For this review, take the finished solid that the model builds, in its own axes (mm). Coordinates: 2 decimals unless noted, no trailing zeros. Loops run counter-clockwise (first coordinate to the right, second up) from the corner with the lowest first, then second, coordinate; pieces in that order, holes last.
1. Take a section at B-B, the plane x = -0.2. Count the separate pieces of the cut face and the enclosed holes in it, then the cut area to 3 significant figures.
2. To check wall thickness, follow probe 1 along Z at (x, y) = (0.4, 15); probe 2 along Y at (x, z) = (-0.75, -85); probe 3 along Y at (x, z) = (0.65, -32.5). State the ranges of each line that lie inside material, in increasing order.
3. Take a section at D-D, the plane z = -68. State the section outline as (x, y) points.
4. Take a section at A-A, the plane z = -22. State the section outline as (x, y) points.
5. Take a section at C-C, the plane y = 57.5. State the section outline as (x, z) points.
6. Clearance check with flat-ended pins moving along their axes: P1, Ø2, axis at x = 0, z = -27, coming from the +Y side; P2, Ø1, axis at x = -1.5, y = 49, coming from the +Z side; P3, Ø2.5, axis at y = 15, z = -85, coming from the -X side; P4, Ø2, axis at x = 1, y = 6.5, coming from the +Z side. State where each tip first meets the part, or that it passes through.
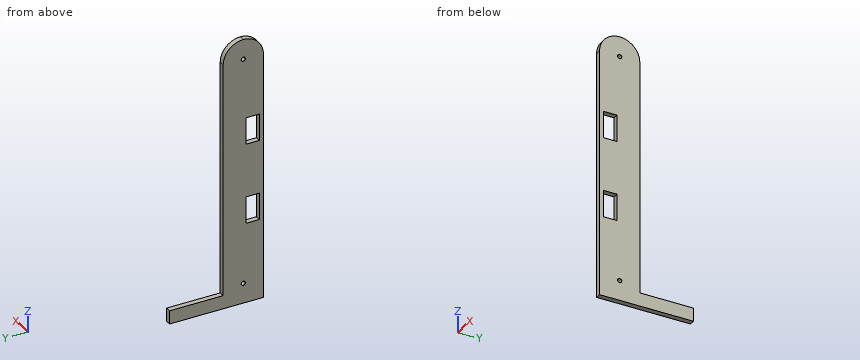
Autodesk Inventor part; units mm, degrees
ref_plane "YZ Plane" through (0, 0, 0) normal (1, 0, 0) x (0, 1, 0)
ref_plane "XZ Plane" through (0, 0, 0) normal (0, 1, 0) x (-1, 0, 0)
ref_plane "XY Plane" through (0, 0, 0) normal (0, 0, 1) x (1, 0, 0)
sketch "Эскиз1" plane through (0, 0, 0) normal (1, 0, 0) x (0, 1, 0)
  line L0 (0, 100) -> (0, -100)
  line L1 (0, -100) -> (30, -100)
  line L2 (30, -100) -> (30, 100)
  line L3 (30, 100) -> (0, 100)
  line L4 (-14, 0) -> (84, 0) construction
  line L5 (0, -140) -> (0, 140) construction
  line L6 (30, -100) -> (70, -100)
  line L7 (70, -100) -> (70, -90)
  line L8 (70, -90) -> (30, -90)
  line L9 (30, -90) -> (30, -100)
  point P0 (0, 0)
  dimension "d0" = 200
  dimension "d1" = 30
  dimension "d2" = 10
  dimension "d3" = 40
extrude "Выдавливание1" add sketch "Эскиз1" along normal mid plane 4
fillet "Сопряжение1" radius 15 2 edges at (0, 30, 100) (0, 0, 100)
sketch "Эскиз2" plane through (2, 0, 0) normal (1, 0, 0) x (0, 0, -1)
  line L0 (-20, 13) -> (-40, 13)
  line L1 (-85, 0) -> (100, 0) construction
  line L2 (100, 0) -> (100, 70)
  line L3 (-40, 13) -> (-20, 13)
  line L4 (-20, 13) -> (-20, 3)
  line L5 (-20, 3) -> (-40, 3)
  line L6 (-40, 3) -> (-40, 13)
  line L7 (20, 13) -> (40, 13)
  line L8 (40, 13) -> (40, 3)
  line L9 (40, 3) -> (20, 3)
  line L10 (20, 3) -> (20, 13)
  point P0 (0, 0)
  point P1 (57.0517, 0.6179)
  dimension "d26" = 10
  dimension "d27" = 20
  dimension "d28" = 3
  dimension "d29" = 20
  dimension "d31" = 20
  dimension "d34" = 3
  dimension "d35" = 10
  dimension "d36" = 20
extrude "Выдавливание2" cut sketch "Эскиз2" against normal blind 4
sketch "Эскиз3" plane through (2, 0, 0) normal (1, 0, 0) x (0, 0, -1)
  arc A0 (-85, 30) -> (-85, 0) centre (-85, 15) ccw
  line L0 (90, 30) -> (-85, 30)
  line L1 (100, 0) -> (100, 70)
  point P0 (0, 0)
  point P1 (85, 15)
  dimension "d16" = 15
  dimension "d17" = 15
hole "Отверстие1" at (2, 15, -85) at (2, 15, 85) direction (-1, 0, 0) diameter 3 depth 4
fillet "Сопряжение2" radius 0.1 4 edges at (2, 15, -83.5) (2, 15, 86.5) (-2, 15, -83.5) (-2, 15, 86.5)
properties part number "Стенка конвейера"
Results list:
1. separate pieces: 1
1. enclosed holes: 4
1. area: 5,890 mm2
2. probe 1: z = -100 to -86.5, -83.5 to 83.5, 86.5 to 100
2. probe 2: y = 0 to 13.5, 16.5 to 30
2. probe 3: y = 0 to 3, 13 to 30
3. outline: (-2, 0) - (2, 0) - (2, 30) - (-2, 30) - close
4. outline: (-2, 0) - (2, 0) - (2, 3) - (-2, 3) - close; (-2, 13) - (2, 13) - (2, 30) - (-2, 30) - close
5. outline: (-2, -100) - (2, -100) - (2, -90) - (-2, -90) - close
6. P1: stops at y = 30
6. P2: stops at z = -90
6. P3: passes through
6. P4: stops at z = 97.99
